The model under review builds one solid part; all positions refer to its coordinate system, in mm. Face numbers are marked on the shaded views. A direction names the side the tool comes from. Round coordinates to 2 decimals unless told otherwise and drop trailing zeros. Write each loop counter-clockwise with the first axis right and the second up, starting at its lowest first coordinate (ties: lowest second). Pieces come first, ordered by that corner, then holes. Notation, with made-up numbers: (34.5, 1) -> (56.5, 1) arc R12 ccw to (56.5, 8) -> close; hole circle Ø4 at (-7.5, 31). An arc over 180 degrees is marked (long way). Answer as a JSON object with one key per item and string values. Group by question number.
1) We need section C-C, the plane y = -5. Write out the cut boundary in (x, z).
2) We need section D-D, the plane y = 18. Write out the cut boundary in (x, z).
3) Insertion check: pin 1 Ø3 at (x, z) = (16, 15.5) entering from -Y; pin 2 Ø5 at (x, y) = (17, 18.5) entering from -Z; pin 3 Ø3 at (x, y) = (18, -25) entering from +Z; pin 4 Ø5 at (x, z) = (78, -26) entering from +Y. Each pin has a flat end and moves straight along its axis. Give the tip position at first contact, or say it passes through.
4) We need section A-A, the plane z = -6. Write out the cut boundary in (x, y).
5) We need section B-B, the plane x = 70. Write out the cut boundary in (y, z), then the cut area to 3 significant figures.
6) To check wall thickness, follow probe 1 along X at (y, z) = (33, -7.5); probe 2 along Z at (x, y) = (24.5, 30); probe 3 along Z at (x, y) = (75, -13.5). State the ranges of each line that lie inside material, in increasing order. Write a range as [from, to].
7) Machinability: for the marked faces 1, 2 and 3, which of the approach directions +Z, -Z, +X, -X, +Y, -Y give a long, thin tool a straight path to every point of the face, cutting with its end or side? Answer none if there is none.
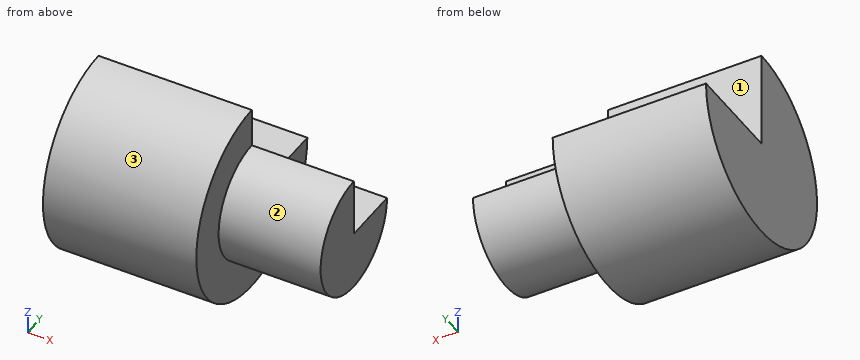
from build123d import *

# Parameters (mm, degrees)
F0_W     = 38.1425693631
F0_H     = 21.7531826347
F1_ANGLE = 270


with BuildPart() as f1:
    # F0 (on Front) → F1 (revolve)
    with BuildSketch(Plane.XZ):
        Polygon((0, 36.3546386361), (0, 0), (57.3628470302, 0), (57.3628470302, 21.7531826347), (57.3628470302, 36.3546386361), align=None)
        with Locations((76.4341317117, 10.8765913174)):
            Rectangle(F0_W, F0_H)
    revolve(axis=Axis((28.6814235151, 0, 0), (1, 0, 0)), revolution_arc=F1_ANGLE)


solid = f1.part
Here are the results:
{
 "1": {"outline": "(0, -36.01) -> (57.36, -36.01) -> (57.36, -21.17) -> (95.51, -21.17) -> (95.51, 21.17) -> (57.36, 21.17) -> (57.36, 36.01) -> (0, 36.01) -> close"},
 "2": {"outline": "(0, -31.59) -> (57.36, -31.59) -> (57.36, -12.21) -> (95.51, -12.21) -> (95.51, 0) -> (0, 0) -> close"},
 "3": {"pin 1": "stops at y = -33.55", "pin 2": "stops at z = -32.64", "pin 3": "stops at z = 27.74", "pin 4": "passes through"},
 "4": {"outline": "(0, -35.86) -> (57.36, -35.86) -> (57.36, -20.91) -> (95.51, -20.91) -> (95.51, 20.91) -> (57.36, 20.91) -> (57.36, 35.86) -> (0, 35.86) -> close"},
 "5": {"outline": "(0, 0) -> (0, 21.75) arc R21.75 ccw (long way) to (21.75, 0) -> close", "area": "1,110 mm^2"},
 "6": {"probe 1": "x = [0, 57.36]", "probe 2": "z = [-20.53, 0]", "probe 3": "z = [-17.06, 17.06]"},
 "7": {"face 1": "+Z, +X, -X, +Y", "face 2": "+X", "face 3": "+X, -X"}
}
